Geometry check sheet. Reference: the model listing, model coordinates, mm. A direction names the side the tool comes from. Round coordinates to 2 decimals unless told otherwise and drop trailing zeros. Write each loop counter-clockwise with the first axis right and the second up, starting at its lowest first coordinate (ties: lowest second). Pieces come first, ordered by that corner, then holes. Notation, with made-up numbers: (62, 69) -> (69, 69) arc R17 cw to (69, 102) -> close; hole circle Ø1 at (-4.5, -8.75). An arc over 180 degrees is marked (long way). Use a Markdown table: item, result.
```python
from build123d import *

# Parameters (mm, degrees)
SKETCH_W  = 24.5
SKETCH_H  = 11.4
PAD_DEPTH = 8.25
FILLET_R  = 2


with BuildPart() as part:
    # Sketch → Pad (new body)
    with BuildSketch(Plane.XY):
        with Locations((12.25, 5.7)):
            Rectangle(SKETCH_W, SKETCH_H)
        Polygon((16.625, 7.95), (17.875, 7.95), (17.875, 6.325), (19.5, 6.325), (19.5, 5.075), (17.875, 5.075), (17.875, 3.45), (16.625, 3.45), (16.625, 5.075), (15, 5.075), (15, 6.325), (16.625, 6.325), align=None, mode=Mode.SUBTRACT)
    extrude(amount=PAD_DEPTH)

    # Fillet
    fillet_edges = [part.edges().sort_by_distance(p)[0] for p in [
        (24.5, 0, 4.125),
        (0, 0, 4.125),
        (24.5, 11.4, 4.125),
        (0, 11.4, 4.125),
    ]]
    fillet(fillet_edges, radius=FILLET_R)


solid = part.part
```
(1) Section check B-B on z = 1.5. Record the cut outline in (x, y) (3 decimals), plus the area to 3 significant figures.
A:
| item | result |
|---|---|
| outline | (0, 2) arc R2 ccw to (2, 0) -> (22.5, 0) arc R2 ccw to (24.5, 2) -> (24.5, 9.4) arc R2 ccw to (22.5, 11.4) -> (2, 11.4) arc R2 ccw to (0, 9.4) -> close; hole (15, 5.075) -> (16.625, 5.075) -> (16.625, 3.45) -> (17.875, 3.45) -> (17.875, 5.075) -> (19.5, 5.075) -> (19.5, 6.325) -> (17.875, 6.325) -> (17.875, 7.95) -> (16.625, 7.95) -> (16.625, 6.325) -> (15, 6.325) -> close |
| area | 266 mm2 |
(2) Access from +Z, -Z, +X, -X, +Y, -Y to the whole of each face (thin tool, end or side, straight path). Record for faces 1 (the face through (16.625, 4, 4)), 2 (the face through (12, 0, 4)).
A:
| item | result |
|---|---|
| face 1 | +Z, -Z |
| face 2 | +Z, -Z, +X, -X, -Y |
(3) Release check for a two-part mould opening along Y. For faces 3 (the face through (12, 11.4, 4)), 4 (the face through (23.9, 0.57, 4.18)), 5 (the face through (15, 6, 4)) record: +Y half, -Y half, draft (parallel to the pull), parting line (faces both ways), or undercut.
A:
| item | result |
|---|---|
| face 3 | +Y half |
| face 4 | -Y half |
| face 5 | undercut |
(4) Section check A-A on x = 19. Record the cut outline in (y, z) (3 decimals), plus the area to 3 significant figures.
A:
| item | result |
|---|---|
| outline | (0, 0) -> (5.075, 0) -> (5.075, 8.25) -> (0, 8.25) -> close; (6.325, 0) -> (11.4, 0) -> (11.4, 8.25) -> (6.325, 8.25) -> close |
| area | 83.7 mm2 |
(5) Thickness scan on line 1 (X direction, y = 4.5, z = 6) (3 decimals); line 2 (X direction, y = 5.5, z = 2.25); line 3 (Y direction, x = 18, z = 6.5) (3 decimals). Record the ranges inside material, lowest first.
A:
| item | result |
|---|---|
| line 1 | x = 0 to 16.625, 17.875 to 24.5 |
| line 2 | x = 0 to 15, 19.5 to 24.5 |
| line 3 | y = 0 to 5.075, 6.325 to 11.4 |
(6) Section check C-C on y = 7.25. Record the cut outline in (x, z) (3 decimals), plus the area to 3 significant figures.
A:
| item | result |
|---|---|
| outline | (0, 0) -> (16.625, 0) -> (16.625, 8.25) -> (0, 8.25) -> close; (17.875, 0) -> (24.5, 0) -> (24.5, 8.25) -> (17.875, 8.25) -> close |
| area | 192 mm2 |
